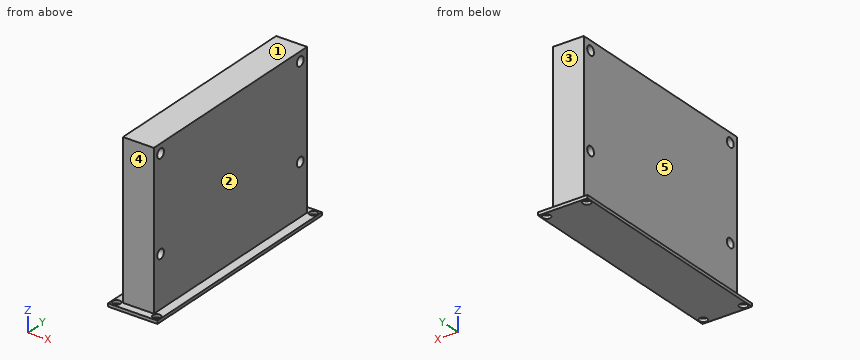
from build123d import *

# Parameters (mm, degrees)
SKETCH080_R     = 1.25
PAD056_DEPTH    = 1
SKETCH081_W     = 10
SKETCH081_H     = 68
PAD057_DEPTH    = 49.5
SKETCH082_R     = 1.5
POCKET015_DEPTH = 13.001


with BuildPart() as part:
    # Sketch080 → Pad056 (new body)
    with BuildSketch(Plane.XY):
        Polygon((-8, 36.5), (8, 36.5), (8, 33), (8, -33), (8, -36.5), (-8, -36.5), (-8, -33), (-8, 33), align=None)
        with Locations((-6.5, 34.75)):
            Circle(SKETCH080_R, mode=Mode.SUBTRACT)
        with Locations((6.5, 34.75)):
            Circle(SKETCH080_R, mode=Mode.SUBTRACT)
        with Locations((-6.5, -34.75)):
            Circle(SKETCH080_R, mode=Mode.SUBTRACT)
        with Locations((6.5, -34.75)):
            Circle(SKETCH080_R, mode=Mode.SUBTRACT)
    extrude(amount=PAD056_DEPTH)

    # Sketch081 (on Face14 of Pad056) → Pad057 (join)
    with BuildSketch(Plane.XY.offset(1)):
        Rectangle(SKETCH081_W, SKETCH081_H)
    extrude(amount=PAD057_DEPTH)

    # Sketch082 (on Face15 of Pad057) → Pocket015 (cut, through all)
    with BuildSketch(Plane(origin=(-5, 0, 0), x_dir=(0, -1, 0), z_dir=(-1, 0, 0))):
        with Locations((31, 47.5)):
            Circle(SKETCH082_R)
        with Locations((-31, 47.5)):
            Circle(SKETCH082_R)
        with Locations((-31, 17.5)):
            Circle(SKETCH082_R)
        with Locations((31, 17.5)):
            Circle(SKETCH082_R)
    extrude(amount=-POCKET015_DEPTH, mode=Mode.SUBTRACT)


with BuildPart() as part_1:
    # Body025 placement: moved
    add(part.part.moved(Location((-15, 0, 47))))


solid = part_1.part
Verification items for the finished model (mm, model axes). Face numbers are marked on the shaded views. A direction names the side the tool comes from. Give positions to 0.01 mm unless a question says otherwise; leave off trailing zeros. Loops run counter-clockwise (first coordinate to the right, second up) from the corner with the lowest first, then second, coordinate; pieces in that order, holes last.
1) Sectioned sample at C-C, the plane x = -11.25. Enter the section's corners in (y, z), then the cut area to 3 significant figures.
2) Thickness scan on line 1 along Y through (x, z) = (-12.25, 64.5); line 2 along Z through (x, y) = (-15, 31); line 3 along Z through (x, y) = (-14.75, -30.5). Record the ranges inside material, lowest first.
3) Sectioned sample at B-B, the plane x = -21.5. Enter the section's corners in (y, z).
4) Sectioned sample at D-D, the plane z = 94.5. Enter the section's corners in (x, y), then the cut area to 3 significant figures.
5) Set-up check for the marked faces 1, 2, 3, 4 and 5: record each of +Z, -Z, +X, -X, +Y, -Y from which the full face is reachable in a straight line by a thin tool's end or side.
6) Depth check by flat-ended pin: pin 1 Ø3 at (y, z) = (-15.5, 54.5) entering from +X; pin 2 Ø8 at (x, z) = (-15, 63) entering from -Y; pin 3 Ø3 at (x, y) = (-21.5, 34.75) entering from +Z. Enter the tip coordinate at first touch or a pass-through.
7) Sectioned sample at A-A, the plane y = 31. Enter the section's corners in (x, z), then the cut area to 3 significant figures.
Answers:
1. outline: (-36.5, 47) - (36.5, 47) - (36.5, 48) - (34, 48) - (34, 97.5) - (-34, 97.5) - (-34, 48) - (-36.5, 48) - close; hole circle Ø3 at (-31, 64.5); hole circle Ø3 at (-31, 94.5); hole circle Ø3 at (31, 64.5); hole circle Ø3 at (31, 94.5)
1. area: 3,410 mm2
2. line 1: y = -34 to -32.5, -29.5 to 29.5, 32.5 to 34
2. line 2: z = 47 to 63, 66 to 93, 96 to 97.5
2. line 3: z = 47 to 63.09, 65.91 to 93.09, 95.91 to 97.5
3. outline: (-36.5, 47) - (-36, 47) - (-36, 48) - (-36.5, 48) - close; (-33.5, 47) - (33.5, 47) - (33.5, 48) - (-33.5, 48) - close; (36, 47) - (36.5, 47) - (36.5, 48) - (36, 48) - close
4. outline: (-20, -34) - (-10, -34) - (-10, -32.5) - (-20, -32.5) - close; (-20, -29.5) - (-10, -29.5) - (-10, 29.5) - (-20, 29.5) - close; (-20, 32.5) - (-10, 32.5) - (-10, 34) - (-20, 34) - close
4. area: 620 mm2
5. face 1: +Z, +X, -X, +Y, -Y
5. face 2: +Z, +X, +Y, -Y
5. face 3: +Z, +X, -X, +Y
5. face 4: +Z, +X, -X, -Y
5. face 5: +Z, -X, +Y, -Y
6. pin 1: stops at x = -10
6. pin 2: stops at y = -34
6. pin 3: stops at z = 48
7. outline: (-23, 47) - (-7, 47) - (-7, 48) - (-10, 48) - (-10, 63) - (-20, 63) - (-20, 48) - (-23, 48) - close; (-20, 66) - (-10, 66) - (-10, 93) - (-20, 93) - close; (-20, 96) - (-10, 96) - (-10, 97.5) - (-20, 97.5) - close
7. area: 451 mm2
